Geometry: final body of the model. Coordinates: model frame, mm. Face numbers are marked on the shaded views. Give positions to 0.01 mm unless a question says otherwise; leave off trailing zeros. Loops run counter-clockwise (first coordinate to the right, second up) from the corner with the lowest first, then second, coordinate; pieces in that order, holes last. Notation, with made-up numbers: (70.25, 71.25) -> (95.25, 71.25) arc R27 cw to (95.25, 105.25) -> close; hole circle Ø1 at (-38.75, 19.25). An arc over 180 degrees is marked (long way). One line per question, with ' | ' between items. Start each with the question number.
Item 1: Section D-D on y = -59. Return loops of the section in (x, z) (3 decimals), then the cut area to 3 significant figures.
Item 2: Section B-B on z = 25. Return loops of the section in (x, y).
Item 3: Section C-C on y = -35. Return loops of the section in (x, z) (3 decimals).
Item 4: Section A-A on x = 53.5. Return loops of the section in (y, z) (3 decimals), then the cut area to 3 significant figures.
Item 5: Mould query, pull axis Y, two halves, no side actions, for the marked faces 1, 2, 3 and 4. Classes: released by +Y, released by -Y, zero draft, split by the parting line, or undercut.
Item 6: Pin query (flat end, axial travel): P1, Ø1, axis at x = -34, z = 6, coming from the +Y side; P2, Ø8, axis at y = -45, z = 12.5, coming from the -X side; P3, Ø3, axis at x = -25.5, z = 8.5, coming from the -Y side. Return the tip coordinate at first contact, or that it passes through.
Item 7: Material intervals for line 1 along Y through (x, z) = (-37, 16.75); line 2 along Z through (x, y) = (60, 1.5) (3 decimals); line 3 along X through (y, z) = (-47, 17.5), sorted ascending. Write a range as [from, to].
from build123d import *

# Parameters (mm, degrees)
F1_W     = 152.4
F1_H     = 88.498586
F1_W_2   = 127
F1_H_2   = 19.05
F2_DEPTH = 3.175
F3_W     = 127
F3_H     = 3.175
F4_DEPTH = 25.4


with BuildPart() as f2:
    # F1 (on face) → F2 (new body)
    with BuildSketch(Plane.XY):
        with Locations((5.21198, -39.078306)):
            Rectangle(F1_W, F1_H)
        with Locations((5.21198, -36.104013)):
            Rectangle(F1_W_2, F1_H_2, mode=Mode.SUBTRACT)
    extrude(amount=F2_DEPTH)

    # F3 (on face) → F4 (join)
    with BuildSketch(Plane.XY.offset(3.175)):
        with Locations((5.21198, -24.991513)):
            Rectangle(F3_W, F3_H)
        with Locations((5.21198, -47.216513)):
            Rectangle(F3_W, F3_H)
    extrude(amount=F4_DEPTH)


solid = f2.part
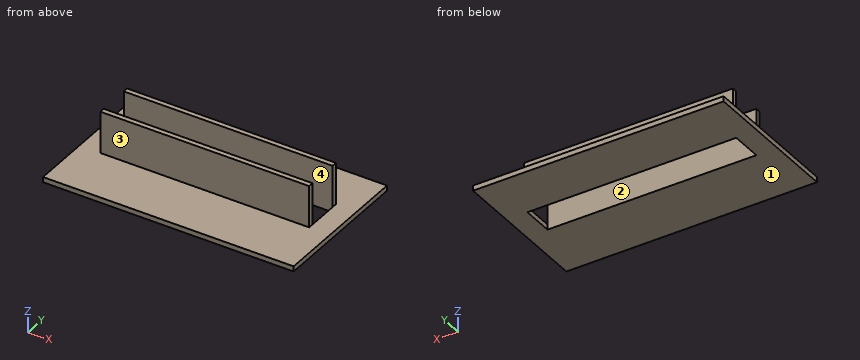
Result sheet:
1) outline: (-70.988, 0) -> (81.412, 0) -> (81.412, 3.175) -> (-70.988, 3.175) -> close | area: 484 mm²
2) outline: (-58.29, -48.8) -> (68.71, -48.8) -> (68.71, -45.63) -> (-58.29, -45.63) -> close; (-58.29, -26.58) -> (68.71, -26.58) -> (68.71, -23.4) -> (-58.29, -23.4) -> close
3) outline: (-70.988, 0) -> (-58.288, 0) -> (-58.288, 3.175) -> (-70.988, 3.175) -> close; (68.712, 0) -> (81.412, 0) -> (81.412, 3.175) -> (68.712, 3.175) -> close
4) outline: (-83.328, 0) -> (-45.629, 0) -> (-45.629, 28.575) -> (-48.804, 28.575) -> (-48.804, 3.175) -> (-83.328, 3.175) -> close; (-26.579, 0) -> (5.171, 0) -> (5.171, 3.175) -> (-23.404, 3.175) -> (-23.404, 28.575) -> (-26.579, 28.575) -> close | area: 382 mm²
5) face 1: zero draft | face 2: undercut | face 3: released by -Y | face 4: undercut
6) P1: stops at y = -23.4 | P2: stops at x = -58.29 | P3: stops at y = -48.8
7) line 1: y = [-48.8, -45.63], [-26.58, -23.4] | line 2: z = [0, 3.175] | line 3: x = [-58.29, 68.71]
